from build123d import *

# Parameters (mm, degrees)
SZKIC1_R                         = 3
DODANIE_WYCI_GNI_CIE1_DEPTH      = 5
SFAZOWANIE1_SIZE                 = 2
SZKIC2_R                         = 12.5
DODANIE_WYCI_GNI_CIE2_DEPTH      = 80
DODANIE_WYCI_GNI_CIE3_DEPTH      = 15
DODANIE_WYCI_GNI_CIE3_DEPTH_BACK = 10
SZKIC5_R                         = 9
SZKIC6_R                         = 8
DODANIE_WYCI_GNI_CIE4_DEPTH      = 10
SZKIC7_R                         = 7
SZKIC7_R_2                       = 5
DODANIE_WYCI_GNI_CIE5_DEPTH      = 2
EBRO1_START                      = -2.5
EBRO1_DEPTH                      = 5
ZAOKR_GLENIE1_R                  = 2.5
DODANIE_WYCI_GNI_CIE6_DEPTH      = 2
DODANIE_WYCI_GNI_CIE6_DEPTH_BACK = 12.5
SZKIC9_R                         = 12.5
OBR_T1_ANGLE                     = 90
SZKIC11_R                        = 8.5
DODANIE_WYCI_GNI_CIE7_DEPTH      = 10
SZKIC12_R                        = 7.5
SZKIC12_R_2                      = 5.5
DODANIE_WYCI_GNI_CIE8_DEPTH      = 2


# Read off the part's stored shape, not the designer's step: Żebro1
with BuildPart() as part:
    # Szkic1 → Dodanie-wyciągnięcie1 (new body)
    with BuildSketch(Plane.XY):
        with BuildLine():
            Line((6, 19.078784028), (6, 25))
            ThreePointArc((6, 25), (0, 31), (-6, 25))
            Line((-6, 25), (-6, 19.078784028))
            ThreePointArc((-6, 19.078784028), (-20, 0), (-6, -19.078784028))
            Line((-6, -19.078784028), (-6, -25))
            ThreePointArc((-6, -25), (0, -31), (6, -25))
            Line((6, -25), (6, -19.078784028))
            ThreePointArc((6, -19.078784028), (20, 0), (6, 19.078784028))
        make_face()
        with Locations((0, 25)):
            Circle(SZKIC1_R, mode=Mode.SUBTRACT)
        with Locations((0, -25)):
            Circle(SZKIC1_R, mode=Mode.SUBTRACT)
    extrude(amount=DODANIE_WYCI_GNI_CIE1_DEPTH)

    # Sfazowanie1
    sfazowanie1_edges = [part.edges().sort_by_distance(p)[0] for p in [
        (20, 0, 5),
        (-20, 0, 5),
    ]]
    chamfer(sfazowanie1_edges, length=SFAZOWANIE1_SIZE)

    # Szkic2 → Dodanie-wyciągnięcie2 (add)
    with BuildSketch(Plane.XY.offset(5)):
        Circle(SZKIC2_R)
    extrude(amount=DODANIE_WYCI_GNI_CIE2_DEPTH)

    # Szkic5 → Dodanie-wyciągnięcie3 (add, two sides: drawn at the far end of the back side and taken through both)
    with BuildSketch(Plane(origin=(0, 12.5, 45), x_dir=(1, 0, 0), z_dir=(0, 0.7071067811865437, -0.7071067811865515)).offset(-DODANIE_WYCI_GNI_CIE3_DEPTH_BACK)):
        with Locations(Location((0, 0, 0), (0, 0, 270))):
            Circle(SZKIC5_R)
    extrude(amount=DODANIE_WYCI_GNI_CIE3_DEPTH + DODANIE_WYCI_GNI_CIE3_DEPTH_BACK)

    # Szkic6 → Dodanie-wyciągnięcie4 (add)
    with BuildSketch(Plane(origin=(0, -5.643398282, 5.643398282), x_dir=(1, 0, 0), z_dir=(0, 0.7071067811865437, -0.7071067811865513))):
        with Locations(Location((0, -40.658639918, 0), (0, 0, 270))):
            Circle(SZKIC6_R)
    extrude(amount=DODANIE_WYCI_GNI_CIE4_DEPTH)

    # Szkic7 → Dodanie-wyciągnięcie5 (add)
    with BuildSketch(Plane(origin=(0, 1.42766953, -1.42766953), x_dir=(1, 0, 0), z_dir=(0, 0.7071067811865437, -0.7071067811865515))):
        with Locations(Location((0, -40.658639918, 0), (0, 0, 270))):
            Circle(SZKIC7_R)
        with Locations(Location((0, -40.658639918, 0), (0, 0, 270))):
            Circle(SZKIC7_R_2, mode=Mode.SUBTRACT)
    extrude(amount=DODANIE_WYCI_GNI_CIE5_DEPTH)

    # Żebro1 outline → Żebro1 (add)
    with BuildSketch(Plane(origin=(0, 0, 0), x_dir=(0, 0, -1), z_dir=(1, 0, 0)).offset(EBRO1_START)):
        with BuildLine():
            Line((-62.727922061, 18.909453225), (-62.727922061, 12))
            Line((-62.727922061, 12), (-42, 12))
            Line((-42, 12), (-42, 26.909453225))
            Line((-42, 26.909453225), (-54.727922061, 26.909453225))
            ThreePointArc((-54.727922061, 26.909453225), (-60.384776311, 24.566307475), (-62.727922061, 18.909453225))
        make_face()
    extrude(amount=EBRO1_DEPTH)

    # Zaokrąglenie1
    zaokr_glenie1_edges = [part.edges().sort_by_distance(p)[0] for p in [
        (-2.5, 15.578450969, 62.727922061),
        (-2.5, 26.909453225, 48.772744048),
        (2.5, 15.578450969, 62.727922061),
        (2.5, 24.566307475, 60.384776311),
        (-2.5, 24.566307475, 60.384776311),
        (2.5, 26.909453225, 48.772744048),
    ]]
    fillet(zaokr_glenie1_edges, radius=ZAOKR_GLENIE1_R - 0.0001)  # a hair under: the kernel refuses the full size

    # Szkic9 → Dodanie-wyciągnięcie6 (add, two sides: drawn at the far end of the back side and taken through both)
    with BuildSketch(Plane(origin=(0, 12.5, 0), x_dir=(1, 0, 0), z_dir=(0, 1, 0)).offset(-DODANIE_WYCI_GNI_CIE6_DEPTH_BACK)):
        with Locations(Location((0, -85, 0), (0, 0, 270))):
            Circle(SZKIC9_R)
    extrude(amount=DODANIE_WYCI_GNI_CIE6_DEPTH + DODANIE_WYCI_GNI_CIE6_DEPTH_BACK)

    # Szkic10 → Obrót1 (revolve)
    with BuildSketch(Plane.XY.offset(85)):
        with BuildLine():
            Line((-12.5, 0), (12.5, 0))
            ThreePointArc((12.5, 0), (0, -12.5), (-12.5, 0))
        make_face()
    revolve(axis=Axis((-12.5, 0, 85), (-1, 0, 0)), revolution_arc=OBR_T1_ANGLE)

    # Szkic11 → Dodanie-wyciągnięcie7 (add)
    with BuildSketch(Plane(origin=(0, 14.5, 0), x_dir=(1, 0, 0), z_dir=(0, 1, 0))):
        with Locations(Location((0, -85, 0), (0, 0, 270))):
            Circle(SZKIC11_R)
    extrude(amount=DODANIE_WYCI_GNI_CIE7_DEPTH)

    # Szkic12 → Dodanie-wyciągnięcie8 (add)
    with BuildSketch(Plane(origin=(0, 24.5, 0), x_dir=(1, 0, 0), z_dir=(0, 1, 0))):
        with Locations(Location((0, -85, 0), (0, 0, 270))):
            Circle(SZKIC12_R)
        with Locations(Location((0, -85, 0), (0, 0, 270))):
            Circle(SZKIC12_R_2, mode=Mode.SUBTRACT)
    extrude(amount=DODANIE_WYCI_GNI_CIE8_DEPTH)


solid = part.part
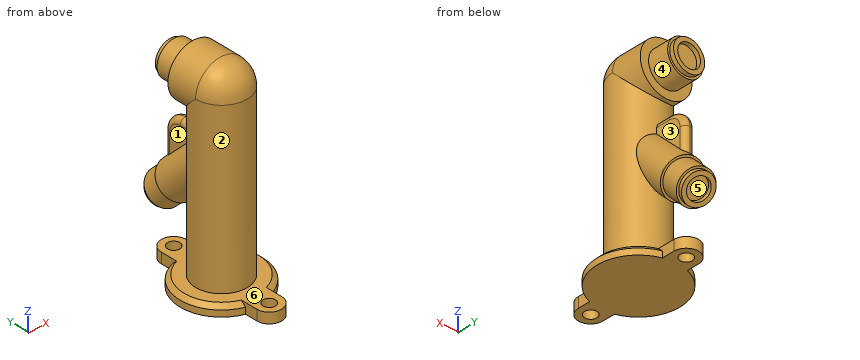
Design review of the part built by this model. Coordinates are the model's own, in mm. Face numbers are marked on the shaded views. A direction names the side the tool comes from. Coordinates: 2 decimals unless noted, no trailing zeros. Order: outer loops, then holes, each group sorted by start corner. A loop starts at its lowest first (then second) coordinate and runs counter-clockwise, first axis right, second up. Notation, with made-up numbers: (4, 18.5) -> (46, 18.5) arc R17 cw to (46, 26.5) -> close; hole circle Ø3 at (82.25, -27.75). An arc over 180 degrees is marked (long way). One line per item, written item: value.
1) Draft analysis for pull direction Y (two halves, no side actions). For the marked faces 5 and 6, state which applies: +Y half, -Y half, draft (parallel to the pull), parting line (faces both ways), or undercut.
Output values:
face 5: undercut
face 6: draft
2) Clearance check with flat-ended pins moving along their axes: P1, Ø12.5, axis at x = -5.5, z = 83, coming from the +Y side; P2, Ø3.5, axis at x = 1.5, z = 84.5, coming from the +Y side; P3, Ø12, axis at x = -15, y = 25.5, coming from the -Z side; P4, Ø5.5, axis at x = 0, y = 25, coming from the +Z side. State where each tip first meets the part, or that it passes through.
Output values:
P1: stops at y = 26.5
P2: stops at y = 24.5
P3: passes through
P4: stops at z = 93.5
3) Machinability: for the marked faces 1, 2, 3 and 4, which of the approach directions +Z, -Z, +X, -X, +Y, -Y give a long, thin tool a straight path to every point of the face, cutting with its end or side? Answer none if there is none.
Output values:
face 1: -X, +Y
face 2: none
face 3: +X, +Y
face 4: +Y
4) We need section A-A, the plane z = 74.5. Give the boundary of the cut face in (x, y), then the cut area to 3 significant figures.
Output values:
outline: (-6.78, 10.5) arc R12.5 ccw (long way) to (6.78, 10.5) -> (6.78, 14.5) -> (-6.78, 14.5) -> close
area: 527 mm2
5) To check wall thickness, follow probe 1 along Y at (x, z) = (0, 1); probe 2 along Y at (x, z) = (1, 22); probe 3 along X at (y, z) = (25.45, 85). State the ranges of each line that lie inside material, in increasing order. Write a range as [from, to].
Output values:
probe 1: y = [-31, -28], [-22, 22], [28, 31]
probe 2: y = [-12.46, 12.46], [24.28, 24.86], [25.7, 27.68]
probe 3: x = [-7.5, -5.5], [5.5, 7.5]
